CAD build for the part. Positions are in the model's coordinates, mm. A direction names the side the tool comes from. Round coordinates to 2 decimals unless told otherwise and drop trailing zeros. Loops run counter-clockwise (first coordinate to the right, second up) from the corner with the lowest first, then second, coordinate; pieces in that order, holes last.
```python
from build123d import *

# Parameters (mm, degrees)
BOSS_EXTRUDE1_DEPTH = 2.5
SKETCH2_R           = 1.6
CUT_EXTRUDE1_DEPTH  = 2.5
SKETCH3_R           = 0.75
CUT_EXTRUDE2_DEPTH  = 2.5
SKETCH4_W           = 6
SKETCH4_H           = 30
CUT_EXTRUDE3_DEPTH  = 10
SKETCH5_R           = 1.5
CUT_EXTRUDE4_DEPTH  = 10
BOSS_EXTRUDE2_DEPTH = 10
SKETCH7_W           = 10
SKETCH7_H           = 1
BOSS_EXTRUDE3_DEPTH = 7
SKETCH8_W           = 56
SKETCH8_H           = 13.315108835
CUT_EXTRUDE5_DEPTH  = 7
FILLET1_R           = 2
CUT_EXTRUDE6_DEPTH  = 7
FILLET3_R           = 2
CUT_EXTRUDE7_DEPTH  = 7
FILLET6_R           = 2
CUT_EXTRUDE8_DEPTH  = 7
FILLET7_R           = 2
CUT_EXTRUDE9_DEPTH  = 7
FILLET8_R           = 2
FILLET9_R           = 2


with BuildPart() as part:
    # Sketch1 → Boss-Extrude1 (new body)
    with BuildSketch(Plane(origin=(0, 0, 0), x_dir=(1, 0, 0), z_dir=(0, 1, 0))):
        Polygon((-10, 33.683794085), (10, 33.683794085), (10, -33.316205915), (-10, -33.316205915), (-26, -14.316205915), (-41, -14.316205915), (-48, -27.316205915), (-59, -38.316205915), (-109, -38.316205915), (-116, -31.316205915), (-116, 31.683794085), (-109, 38.683794085), (-59, 38.683794085), (-48, 27.683794085), (-41, 14.683794085), (-26, 14.683794085), align=None)
    extrude(amount=BOSS_EXTRUDE1_DEPTH)

    # Sketch2 → Cut-Extrude1 (cut)
    with BuildSketch(Plane(origin=(0, 2.5, 0), x_dir=(1, 0, 0), z_dir=(0, 1, 0))):
        with Locations(Location((6.8, 18.933794085, 0), (0, 0, 270))):
            Circle(SKETCH2_R)
        with Locations(Location((6.8, -18.566205915, 0), (0, 0, 270))):
            Circle(SKETCH2_R)
    extrude(amount=-CUT_EXTRUDE1_DEPTH, mode=Mode.SUBTRACT)

    # Sketch3 → Cut-Extrude2 (cut)
    with BuildSketch(Plane(origin=(0, 2.5, 0), x_dir=(1, 0, 0), z_dir=(0, 1, 0))):
        with Locations(Location((-107, 33.183794085, 0), (0, 0, 270))):
            Circle(SKETCH3_R)
        with Locations(Location((-61, 33.183794085, 0), (0, 0, 270))):
            Circle(SKETCH3_R)
        with Locations(Location((-61, -32.816205915, 0), (0, 0, 270))):
            Circle(SKETCH3_R)
        with Locations(Location((-107, -32.816205915, 0), (0, 0, 270))):
            Circle(SKETCH3_R)
    extrude(amount=-CUT_EXTRUDE2_DEPTH, mode=Mode.SUBTRACT)

    # Sketch4 → Cut-Extrude3 (cut)
    with BuildSketch(Plane(origin=(0, 2.5, 0), x_dir=(1, 0, 0), z_dir=(0, 1, 0))):
        with Locations((7, 0.183794085)):
            Rectangle(SKETCH4_W, SKETCH4_H)
    extrude(amount=-CUT_EXTRUDE3_DEPTH, mode=Mode.SUBTRACT)

    # Sketch5 → Cut-Extrude4 (cut)
    with BuildSketch(Plane(origin=(0, 2.5, 0), x_dir=(1, 0, 0), z_dir=(0, 1, 0))):
        with Locations(Location((-87, 22.683794085, 0), (0, 0, 270))):
            Circle(SKETCH5_R)
        with Locations(Location((-61.5, 22.683794085, 0), (0, 0, 270))):
            Circle(SKETCH5_R)
        with Locations(Location((-61.5, -22.316205915, 0), (0, 0, 270))):
            Circle(SKETCH5_R)
        with Locations(Location((-87, -22.316205915, 0), (0, 0, 270))):
            Circle(SKETCH5_R)
    extrude(amount=-CUT_EXTRUDE4_DEPTH, mode=Mode.SUBTRACT)

    # Sketch6 → Boss-Extrude2 (add)
    with BuildSketch(Plane(origin=(0, 2.5, 0), x_dir=(1, 0, 0), z_dir=(0, 1, 0))):
        Polygon((4, -11.63131475), (-62, -11.63131475), (-62, -4.63131475), (-60, -4.63131475), (-60, -9.63131475), (2, -9.63131475), (2, 9.683794085), (-60, 9.683794085), (-60, 11.683794085), (4, 11.683794085), align=None)
    extrude(amount=BOSS_EXTRUDE2_DEPTH)

    # Sketch7 → Boss-Extrude3 (add)
    with BuildSketch(Plane(origin=(0, 2.5, 0), x_dir=(1, 0, 0), z_dir=(0, 1, 0))):
        with Locations((-74.25, 7.183794085)):
            Rectangle(SKETCH7_W, SKETCH7_H)
        with Locations((-74.25, -6.816205915)):
            Rectangle(SKETCH7_W, SKETCH7_H)
    extrude(amount=BOSS_EXTRUDE3_DEPTH)

    # Sketch8 → Cut-Extrude5 (cut)
    with BuildSketch(Plane(origin=(0, 2.5, 0), x_dir=(1, 0, 0), z_dir=(0, 1, 0))):
        with Locations((-29, 0.026239668)):
            Rectangle(SKETCH8_W, SKETCH8_H)
    extrude(amount=-CUT_EXTRUDE5_DEPTH, mode=Mode.SUBTRACT)

    # Fillet1
    fillet1_edges = [part.edges().sort_by_distance(p)[0] for p in [
        (-10, 1.25, 33.316205915),
        (-26, 1.25, 14.316205915),
        (-41, 1.25, 14.316205915),
        (-48, 1.25, 27.316205915),
        (-59, 1.25, 38.316205915),
        (-109, 1.25, 38.316205915),
        (-116, 1.25, 31.316205915),
        (-116, 1.25, -31.683794085),
        (-109, 1.25, -38.683794085),
        (-59, 1.25, -38.683794085),
        (-48, 1.25, -27.683794085),
        (-41, 1.25, -14.683794085),
        (-26, 1.25, -14.683794085),
        (-10, 1.25, -33.683794085),
    ]]
    fillet(fillet1_edges, radius=FILLET1_R)

    # Sketch9 → Cut-Extrude6 (cut)
    with BuildSketch(Plane(origin=(0, 2.5, 0), x_dir=(1, 0, 0), z_dir=(0, 1, 0))):
        Polygon((-79.25, 3.683794085), (-79.25, -3.316205915), (-69.25, -3.316205915), (-67.358162245, -6.816205915), (-63.608162245, -6.816205915), (-63.608162245, 7.183794085), (-67.358162245, 7.183794085), (-69.25, 3.683794085), align=None)
    extrude(amount=-CUT_EXTRUDE6_DEPTH, mode=Mode.SUBTRACT)

    # Fillet3
    fillet3_edges = [part.edges().sort_by_distance(p)[0] for p in [
        (-79.25, 1.25, -3.683794085),
        (-69.25, 1.25, -3.683794085),
        (-67.358162245, 1.25, -7.183794085),
        (-63.608162245, 1.25, -7.183794085),
        (-63.608162245, 1.25, 6.816205915),
        (-67.358162245, 1.25, 6.816205915),
        (-69.25, 1.25, 3.316205915),
        (-79.25, 1.25, 3.316205915),
    ]]
    fillet(fillet3_edges, radius=FILLET3_R)

    # Sketch10 → Cut-Extrude7 (cut)
    with BuildSketch(Plane(origin=(0, 2.5, 0), x_dir=(1, 0, 0), z_dir=(0, 1, 0))):
        Polygon((-44, -14.13131475), (-56, -14.13131475), (-56, -31.14037523), align=None)
        Polygon((-44, 14.183794085), (-56, 14.183794085), (-56, 32.891774512), align=None)
    extrude(amount=-CUT_EXTRUDE7_DEPTH, mode=Mode.SUBTRACT)

    # Fillet6
    fillet6_edges = [part.edges().sort_by_distance(p)[0] for p in [
        (-44, 1.25, 14.13131475),
        (-56, 1.25, 31.14037523),
        (-56, 1.25, 14.13131475),
        (-56, 1.25, -32.891774512),
        (-44, 1.25, -14.183794085),
        (-56, 1.25, -14.183794085),
    ]]
    fillet(fillet6_edges, radius=FILLET6_R)

    # Sketch11 → Cut-Extrude8 (cut)
    with BuildSketch(Plane(origin=(0, 2.5, 0), x_dir=(1, 0, 0), z_dir=(0, 1, 0))):
        Polygon((-4.220314933, 29.952266722), (-9.220314933, 29.952266722), (-21.314371027, 15.59057511), (0.685628973, 15.59057511), align=None)
        Polygon((-20.861245147, -14.911119692), (1.138754853, -14.911119692), (-2.563588823, -30.702086576), (-7.563588823, -30.702086576), align=None)
    extrude(amount=-CUT_EXTRUDE8_DEPTH, mode=Mode.SUBTRACT)

    # Fillet7
    fillet7_edges = [part.edges().sort_by_distance(p)[0] for p in [
        (-4.220314933, 1.25, -29.952266722),
        (0.685628973, 1.25, -15.59057511),
        (-21.314371027, 1.25, -15.59057511),
        (-9.220314933, 1.25, -29.952266722),
        (-7.563588823, 1.25, 30.702086576),
        (-20.861245147, 1.25, 14.911119692),
        (1.138754853, 1.25, 14.911119692),
        (-2.563588823, 1.25, 30.702086576),
    ]]
    fillet(fillet7_edges, radius=FILLET7_R)

    # Sketch12 → Cut-Extrude9 (cut)
    with BuildSketch(Plane(origin=(0, 2.5, 0), x_dir=(1, 0, 0), z_dir=(0, 1, 0))):
        Polygon((-112, 28.683794085), (-112, 2.683794085), (-89, 2.683794085), align=None)
        Polygon((-112, -2.316205915), (-112, -28.316205915), (-89, -2.316205915), align=None)
    extrude(amount=-CUT_EXTRUDE9_DEPTH, mode=Mode.SUBTRACT)

    # Fillet8
    fillet8_edges = [part.edges().sort_by_distance(p)[0] for p in [
        (-112, 1.25, -28.683794085),
        (-89, 1.25, -2.683794085),
        (-112, 1.25, -2.683794085),
        (-112, 1.25, 2.316205915),
        (-89, 1.25, 2.316205915),
        (-112, 1.25, 28.316205915),
    ]]
    fillet(fillet8_edges, radius=FILLET8_R)

    # Fillet9
    fillet9_edges = [part.edges().sort_by_distance(p)[0] for p in [
        (-57, 1.25, 6.63131475),
        (-57, 1.25, -6.683794085),
        (-1, 1.25, -6.683794085),
        (-1, 1.25, 6.63131475),
    ]]
    fillet(fillet9_edges, radius=FILLET9_R)


solid = part.part
```
Item 1: 3-axis set-ups, long thin cutter, end or side, ignore diameter. For faces 1 (the flat face through (-102, 1, 2.316)), 2 (the flat face through (0, 1, -33.684)), 3 (the flat face through (7, 1, -15.184)): which of +Z, -Z, +X, -X, +Y, -Y reach the whole face in a straight line?
Answers follow:
face 1: +Y, -Y
face 2: -Z, +X, +Y, -Y
face 3: +X, +Y, -Y
Item 2: Cut at B-B, the plane y = 7. Give the cut face in (x, z).
Answers follow:
outline: (-79.25, -7.68) - (-69.25, -7.68) - (-69.25, -6.68) - (-79.25, -6.68) - close; (-79.25, 6.32) - (-69.25, 6.32) - (-69.25, 7.32) - (-79.25, 7.32) - close; (-62, 4.63) - (-60, 4.63) - (-60, 9.63) - (2, 9.63) - (2, -9.68) - (-60, -9.68) - (-60, -11.68) - (4, -11.68) - (4, 11.63) - (-62, 11.63) - close
Item 3: Flat gauge pins, fed straight in: P1, Ø1, axis at x = -55, y = 8, coming from the +Z side; P2, Ø1.1, axis at y = 5.5, z = -7.5, coming from the +X side; P3, Ø2, axis at x = -23.5, z = 7.5, coming from the +Y side; P4, Ø1.2, axis at x = -107, z = -33.18, coming from the +Y side. Where does each tip first touch, or does it go through?
Answers follow:
P1: stops at z = 11.63
P2: stops at x = 4
P3: stops at y = 2.5
P4: passes through
Item 4: Cut at A-A, the plane x = -87. Give the cut face in (y, z), plus the area to 4 significant figures.
Answers follow:
outline: (0, -38.68) - (2.5, -38.68) - (2.5, -24.18) - (0, -24.18) - close; (0, -21.18) - (2.5, -21.18) - (2.5, 20.82) - (0, 20.82) - close; (0, 23.82) - (2.5, 23.82) - (2.5, 38.32) - (0, 38.32) - close
area: 177.5 mm2
Item 5: Two-plate mould, pull along X, no slides. Class faces 4 (the flat face through (-74, 6, 7.316)), 5 (the cylindrical face through (-54.571, 1.232, 26.753)), 6 (the cylindrical face through (-110.74, 1.232, -25.262)), 7 (the flat face through (4, 6, 0)): released by +X, released by -X, zero draft, split by the parting line, or undercut.
Answers follow:
face 4: zero draft
face 5: undercut
face 6: undercut
face 7: released by +X
Item 6: Probe line 1 (Z direction, x = -61, y = 0.5); line 2 (Z direction, x = -32, y = 8); line 3 (Z direction, x = -107, y = 1.8). List the from-to ranges inside material, lowest first.
Answers follow:
line 1: z = -38.68 to -33.93, -32.43 to -24.1, -21.27 to 20.9, 23.73 to 32.07, 33.57 to 38.32
line 2: z = -11.68 to -9.68, 9.63 to 11.63
line 3: z = -38.68 to -33.93, -32.43 to -23.03, -2.68 to 2.32, 22.66 to 32.07, 33.57 to 38.32
Item 7: Cut at C-C, the plane x = 6.8. Give the cut face in (y, z), plus the area to 3 significant figures.
Answers follow:
outline: (0, -33.68) - (2.5, -33.68) - (2.5, -20.53) - (0, -20.53) - close; (0, -17.33) - (2.5, -17.33) - (2.5, -15.18) - (0, -15.18) - close; (0, 14.82) - (2.5, 14.82) - (2.5, 16.97) - (0, 16.97) - close; (0, 20.17) - (2.5, 20.17) - (2.5, 33.32) - (0, 33.32) - close
area: 76.5 mm2
